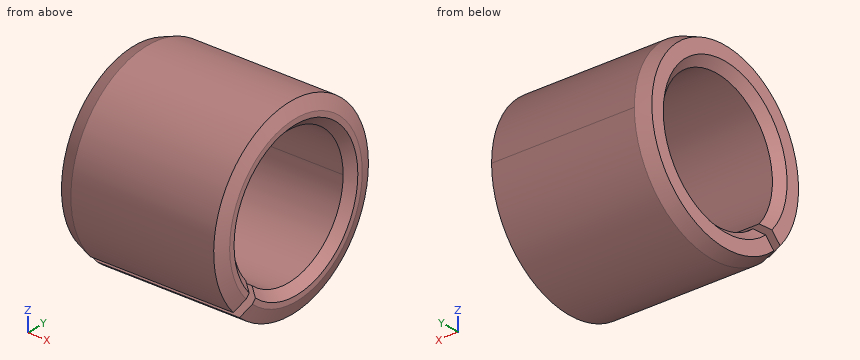
```python
from build123d import *

# Parameters (mm, degrees)
SKETCH1_W             = 6
SKETCH1_H             = 3.5
CUT_EXTRUDE1_DEPTH    = 7
SKETCH3_W             = 6
SKETCH3_H             = 2.5
CHAMFER1_SIZE         = 0.3
CHAMFER2_SIZE         = 0.181985117
CHAMFER2_SIZE2        = 0.5
CHAMFER2_PART_2_SIZE  = 0.181985117
CHAMFER2_PART_2_SIZE2 = 0.5


with BuildPart() as part:
    # Sketch1 → Revolve1 (revolve)
    with BuildSketch(Plane.XY):
        with Locations((3, 1.75)):
            Rectangle(SKETCH1_W, SKETCH1_H)
    revolve(axis=Axis((0, 0, 0), (1, 0, 0)))

    # Sketch2 → Cut-Extrude1 (cut, through all)
    with BuildSketch(Plane.ZY):
        with BuildLine():
            Line((-2.329408464, -2.612251176), (-1.620679662, -1.903522375))
            ThreePointArc((-1.620679662, -1.903522375), (-1.767766953, -1.767766953), (-1.903522375, -1.620679662))
            Line((-1.903522375, -1.620679662), (-2.612251176, -2.329408464))
            ThreePointArc((-2.612251176, -2.329408464), (-2.474873734, -2.474873734), (-2.329408464, -2.612251176))
        make_face()
    extrude(amount=-CUT_EXTRUDE1_DEPTH, mode=Mode.SUBTRACT)

    # Sketch3 → Cut-Revolve1 (revolve, cut)
    with BuildSketch(Plane.XY):
        with Locations((3, 1.25)):
            Rectangle(SKETCH3_W, SKETCH3_H)
    revolve(axis=Axis((0, 0, 0), (1, 0, 0)), mode=Mode.SUBTRACT)

    # Chamfer1
    chamfer1_edges = [part.edges().sort_by_distance(p)[0] for p in [
        (0, -0.863479607, 2.346146408),
        (6, -0.863479607, 2.346146408),
    ]]
    chamfer(chamfer1_edges, length=CHAMFER1_SIZE)

    # Chamfer2
    chamfer2_edges = [part.edges().sort_by_distance(p)[0] for p in [
        (0, -1.246419047, 3.270541172),
    ]]
    chamfer2_side = [part.faces().sort_by_distance(p)[0] for p in [
        (0, -2.011414437, -2.434257149),
    ]]
    chamfer(chamfer2_edges, length=CHAMFER2_SIZE, length2=CHAMFER2_SIZE2, reference=chamfer2_side[0])

    # Chamfer2 part 2
    chamfer2_part_2_edges = [part.edges().sort_by_distance(p)[0] for p in [
        (6, -1.246419047, 3.270541172),
    ]]
    chamfer2_part_2_side = [part.faces().sort_by_distance(p)[0] for p in [
        (3, -1.246419047, 3.270541172),
    ]]
    chamfer(chamfer2_part_2_edges, length=CHAMFER2_PART_2_SIZE, length2=CHAMFER2_PART_2_SIZE2, reference=chamfer2_part_2_side[0])


solid = part.part
```
The model under review builds one solid part; all positions refer to its coordinate system, in mm. Give positions to 0.01 mm unless a question says otherwise; leave off trailing zeros. Loops run counter-clockwise (first coordinate to the right, second up) from the corner with the lowest first, then second, coordinate; pieces in that order, holes last. Notation, with made-up numbers: (-3, 7.25) -> (30, 7.25) arc R13 cw to (30, 32.25) -> close; hole circle Ø2 at (34.25, 6). An arc over 180 degrees is marked (long way). Use CSV: the item, a comma, the result in double quotes.
1. For P1, Ø1.5, axis at x = 1.5, y = -2.5, coming from the -Z side; P2, Ø4, axis at y = 0, z = 0, coming from the -X side; P3, Ø1, axis at y = 1.5, z = 1.5, coming from the -X side, all flat-tipped, find the tip position at first contact; note any pin that passes through.
Result:
P1,"stops at z = -3.03"
P2,"passes through"
P3,"stops at x = 0.18"
2. Consider section B-B, the plane x = 2.5. Write out the cut boundary in (y, z), then the cut area to 3 significant figures.
Result:
outline,"(-2.61, -2.33) -> (-1.9, -1.62) arc R2.5 cw (long way) to (-1.62, -1.9) -> (-2.33, -2.61) arc R3.5 ccw (long way) to start"
area,"18.4 mm²"
3. To check wall thickness, follow probe 1 along Z at (x, y) = (2.1, 0); probe 2 along Z at (x, y) = (2.25, -0.75). State the ranges of each line that lie inside material, in increasing order. Write a range as from..to.
Result:
probe 1,"z = -3.5..-2.5, 2.5..3.5"
probe 2,"z = -3.42..-2.38, 2.38..3.42"
4. Consider section A-A, the plane y = 0. Write out the cut boundary in (x, z), then the cut area to 3 significant figures.
Result:
outline,"(0, -3.32) -> (0.5, -3.5) -> (5.82, -3.5) -> (6, -3) -> (6, -2.8) -> (5.7, -2.5) -> (0.3, -2.5) -> (0, -2.8) -> close; (0, 2.8) -> (0.3, 2.5) -> (5.7, 2.5) -> (6, 2.8) -> (6, 3) -> (5.82, 3.5) -> (0.5, 3.5) -> (0, 3.32) -> close"
area,"11.6 mm²"
